Part model, mm, in its own coordinate system. A direction names the side the tool comes from. Round coordinates to 2 decimals unless told otherwise and drop trailing zeros. Write each loop counter-clockwise with the first axis right and the second up, starting at its lowest first coordinate (ties: lowest second). Pieces come first, ordered by that corner, then holes. Notation, with made-up numbers: (-36.75, 1.5) -> (-24.75, 1.5) arc R18 cw to (-24.75, 7.5) -> close; hole circle Ø8 at (-18.5, 0.5). An arc over 180 degrees is marked (long way). Return JSON: item names as keys, results as strings. Group by question number.
```python
from build123d import *

# Parameters (mm, degrees)
BOSS_EXTRU_1_DEPTH      = 5
ENL_V_MAT_EXTRU_1_DEPTH = 55.313902456
ESQUISSE3_R             = 2.5
ENL_V_MAT_EXTRU_2_DEPTH = 55.313902456


with BuildPart() as part:
    # Esquisse1 → Boss.-Extru.1 (new body)
    with BuildSketch(Plane.XY):
        with BuildLine():
            Line((28, -45), (-28, -45))
            ThreePointArc((-28, -45), (-29.414213562, -44.414213562), (-30, -43))
            Line((-30, -43), (-30, 43))
            ThreePointArc((-30, 43), (-29.414213562, 44.414213562), (-28, 45))
            Line((-28, 45), (28, 45))
            ThreePointArc((28, 45), (29.414213562, 44.414213562), (30, 43))
            Line((30, 43), (30, -43))
            ThreePointArc((30, -43), (29.414213562, -44.414213562), (28, -45))
        make_face()
    extrude(amount=BOSS_EXTRU_1_DEPTH)

    # Esquisse2 → Enlèv. mat.-Extru.1 (cut, through all)
    with BuildSketch(Plane(origin=(0, 0, 0), x_dir=(-1, 0, 0), z_dir=(0, 0, -1))):
        with BuildLine():
            Line((18, -27.5), (-18, -27.5))
            ThreePointArc((-18, -27.5), (-19.414213562, -26.914213562), (-20, -25.5))
            Line((-20, -25.5), (-20, 25.5))
            ThreePointArc((-20, 25.5), (-19.414213562, 26.914213562), (-18, 27.5))
            Line((-18, 27.5), (18, 27.5))
            ThreePointArc((18, 27.5), (19.414213562, 26.914213562), (20, 25.5))
            Line((20, 25.5), (20, -25.5))
            ThreePointArc((20, -25.5), (19.414213562, -26.914213562), (18, -27.5))
        make_face()
    extrude(amount=-ENL_V_MAT_EXTRU_1_DEPTH, mode=Mode.SUBTRACT)

    # Esquisse3 → Enlèv. mat.-Extru.2 (cut, through all)
    with BuildSketch(Plane.XY.offset(5)):
        with Locations((-22.5, -39.5)):
            Circle(ESQUISSE3_R)
        with Locations((22.5, -39.5)):
            Circle(ESQUISSE3_R)
        with Locations((-22.5, 39.5)):
            Circle(ESQUISSE3_R)
        with Locations((22.5, 39.5)):
            Circle(ESQUISSE3_R)
    extrude(amount=-ENL_V_MAT_EXTRU_2_DEPTH, mode=Mode.SUBTRACT)


solid = part.part
```
Item 1: Cut at A-A (x = -22.5). Write the cut outline in (y, z), then the cut area to 3 significant figures.
Item 2: Cut at B-B (y = 21). Write the cut outline in (x, z).
Item 3: Wall check: L1, parallel to Y at x = 22.5, z = 2.45; L2, parallel to Y at x = 5.5, z = 1.6; L3, parallel to X at y = -19.5, z = 4.2. Give the ranges that are in metal, low to high.
Item 4: Cut at C-C (z = 2.45). Write the cut outline in (x, y), then the cut area to 3 significant figures.
Item 5: Which spindle directions (+Z, -Z, +X, -X, +Y, -Y) get a long thin tool onto all of the face, cutting with end or side? Do faces 1 (the face through (0, 27.5, 2)), 2 (the face through (-29.4, -44.43, 2.46)). Say none if no direction does.
Item 6: Flat gauge pin, fed straight in: P1, Ø6, axis at x = 22.5, y = -39.5, coming from the +Z side. Where does the tip first touch, or does it go through?
Item 7: Two-plate mould, pull along Y, no slides. Class faces 3 (the face through (-24.5, 38, 2.5)), 4 (the face through (0, -27.5, 2)), 5 (the face through (20.4, 0.6, 0)), 6 (the face through (-29.43, 44.4, 2.46)): released by +Y, released by -Y, zero draft, split by the parting line, or undercut.
Item 8: Cut at D-D (y = -39.5). Write the cut outline in (x, z).
Checks:
{
 "1": {"outline": "(-45, 0) -> (-42, 0) -> (-42, 5) -> (-45, 5) -> close; (-37, 0) -> (37, 0) -> (37, 5) -> (-37, 5) -> close; (42, 0) -> (45, 0) -> (45, 5) -> (42, 5) -> close", "area": "400 mm2"},
 "2": {"outline": "(-30, 0) -> (-20, 0) -> (-20, 5) -> (-30, 5) -> close; (20, 0) -> (30, 0) -> (30, 5) -> (20, 5) -> close"},
 "3": {"L1": "y = -45 to -42, -37 to 37, 42 to 45", "L2": "y = -45 to -27.5, 27.5 to 45", "L3": "x = -30 to -20, 20 to 30"},
 "4": {"outline": "(-30, -43) arc R2 ccw to (-28, -45) -> (28, -45) arc R2 ccw to (30, -43) -> (30, 43) arc R2 ccw to (28, 45) -> (-28, 45) arc R2 ccw to (-30, 43) -> close; hole circle Ø5 at (-22.5, -39.5); hole circle Ø5 at (-22.5, 39.5); hole (-20, -25.5) arc R2 ccw to (-18, -27.5) -> (18, -27.5) arc R2 ccw to (20, -25.5) -> (20, 25.5) arc R2 ccw to (18, 27.5) -> (-18, 27.5) arc R2 ccw to (-20, 25.5) -> close; hole circle Ø5 at (22.5, -39.5); hole circle Ø5 at (22.5, 39.5)", "area": "3,120 mm2"},
 "5": {"face 1": "+Z, -Z", "face 2": "+Z, -Z, -X, -Y"},
 "6": {"P1": "stops at z = 5"},
 "7": {"face 3": "undercut", "face 4": "undercut", "face 5": "zero draft", "face 6": "released by +Y"},
 "8": {"outline": "(-30, 0) -> (-25, 0) -> (-25, 5) -> (-30, 5) -> close; (-20, 0) -> (20, 0) -> (20, 5) -> (-20, 5) -> close; (25, 0) -> (30, 0) -> (30, 5) -> (25, 5) -> close"}
}
